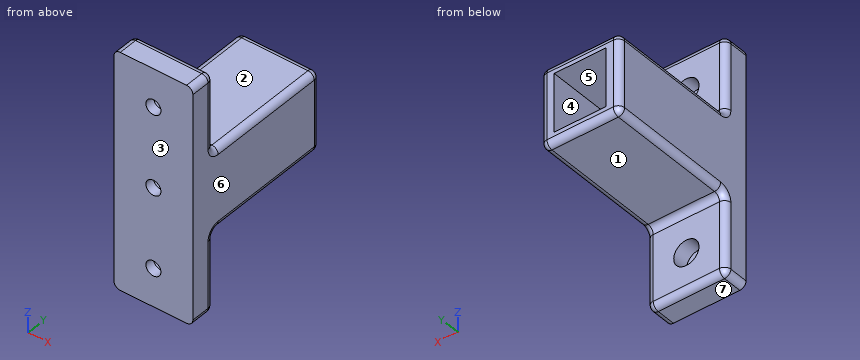
from build123d import *

# Parameters (mm, degrees)
SKETCH1_W               = 25
SKETCH1_H               = 25
SKETCH1_W_2             = 16.4
SKETCH1_H_2             = 18.5
BOSS_EXTRUDE1_DEPTH     = 50
SKETCH6_W               = 25
SKETCH6_H               = 75
BOSS_EXTRUDE3_DEPTH     = 8
FILLET2_R               = 2
SKETCH7_R               = 4
CUT_EXTRUDE1_DEPTH      = 5
CUT_EXTRUDE4_DEPTH      = 64.73774392
CUT_EXTRUDE4_DEPTH_BACK = 64.73774392
SKETCH8_R               = 2.38125


with BuildPart() as part:
    # Sketch1 → Boss-Extrude1 (new body)
    with BuildSketch(Plane(origin=(0, 0, 0), x_dir=(1, 0, 0), z_dir=(0, 1, 0))):
        Rectangle(SKETCH1_W, SKETCH1_H)
        Rectangle(SKETCH1_W_2, SKETCH1_H_2, mode=Mode.SUBTRACT)
    extrude(amount=BOSS_EXTRUDE1_DEPTH)

    # Sketch6 → Boss-Extrude3 (add)
    with BuildSketch(Plane(origin=(0, 0, 0), x_dir=(1, 0, 0), z_dir=(0, 1, 0))):
        Rectangle(SKETCH6_W, SKETCH6_H)
    extrude(amount=BOSS_EXTRUDE3_DEPTH)

    # Fillet2
    fillet2_edges = [part.edges().sort_by_distance(p)[0] for p in [
        (-12.5, 50, 0),
        (0, 50, 12.5),
        (12.5, 4, 37.5),
        (-12.5, 4, -37.5),
        (-12.5, 8, -25),
        (0, 8, -12.5),
        (12.5, 8, -25),
        (0, 8, -37.5),
        (12.5, 8, 25),
        (0, 8, 12.5),
        (-12.5, 8, 25),
        (0, 8, 37.5),
        (12.5, 4, -37.5),
        (-12.5, 4, 37.5),
        (12.5, 50, 0),
        (12.5, 29, 12.5),
        (-12.5, 29, 12.5),
        (-12.5, 29, -12.5),
        (12.5, 29, -12.5),
        (0, 50, -12.5),
    ]]
    fillet(fillet2_edges, radius=FILLET2_R)

    # Sketch7 → Cut-Extrude1 (cut)
    with BuildSketch(Plane(origin=(0, 8, 0), x_dir=(1, 0, 0), z_dir=(0, 1, 0))):
        with Locations(Location((0, 0, 0), (0, 0, 270))):
            Circle(SKETCH7_R)
        with Locations(Location((0, 25.4, 0), (0, 0, 270))):
            Circle(SKETCH7_R)
        with Locations(Location((0, -25.4, 0), (0, 0, 270))):
            Circle(SKETCH7_R)
    extrude(amount=-CUT_EXTRUDE1_DEPTH, mode=Mode.SUBTRACT)

    # Sketch8 → Cut-Extrude4 (cut, two sides: drawn at the far end of the back side and taken through both)
    with BuildSketch(Plane(origin=(0, 0, 0), x_dir=(1, 0, 0), z_dir=(0, 1, 0)).offset(-CUT_EXTRUDE4_DEPTH_BACK)):
        with Locations(Location((0, 0, 0), (0, 0, 270))):
            Circle(SKETCH8_R)
        with Locations(Location((0, 25.4, 0), (0, 0, 270))):
            Circle(SKETCH8_R)
        with Locations(Location((0, -25.4, 0), (0, 0, 270))):
            Circle(SKETCH8_R)
    extrude(amount=CUT_EXTRUDE4_DEPTH + CUT_EXTRUDE4_DEPTH_BACK, mode=Mode.SUBTRACT)


solid = part.part
CAD build for the part. Positions are in the model's coordinates, mm. Face numbers are marked on the shaded views. A direction names the side the tool comes from. Coordinates: 2 decimals unless noted, no trailing zeros. Loops run counter-clockwise (first coordinate to the right, second up) from the corner with the lowest first, then second, coordinate; pieces in that order, holes last. Notation, with made-up numbers: (-1, -19) - (57, -19) arc R21 cw to (57, 19) - close; hole circle Ø6 at (-22, 2). An arc over 180 degrees is marked (long way). Use one line per item in the form item = value. Start each with the question number.
1) Band-saw the part on A-A (y = 24). Give the cut face in (x, z), and give its area (3 significant figures).
2) Band-saw the part on B-B (z = 0). Give the cut face in (x, y).
3) Two-plate mould, pull along X, no slides. Class the marked faces 4, 5, 6 and 7: +X half, -X half, draft (parallel to the pull), parting line (faces both ways), or undercut.
4) Tool access for the marked faces 1, 2 and 3: list every direction of +Z, -Z, +X, -X, +Y, -Y with a clear straight run to the whole face (end or side of a thin tool).
5) Band-saw the part on D-D (z = -18.5). Give the cut face in (x, y), and give its area (3 significant figures).
6) Flat gauge pins, fed straight in: pin 1 (2 mm diameter, centred on x = 7.5, y = 30, fed in from +Z); pin 2 (5 mm diameter, centred on x = 2.5, y = 27, fed in from -Z); pin 3 (6.5 mm diameter, centred on x = -1.5, z = -26, fed in from +Y). Where does each tip first touch, or does it go through?
7) Band-saw the part on C-C (x = 7.25). Give the cut face in (y, z), and give its area (3 significant figures).
8) Drill centre lines: L1, parallel to X at y = 29.5, z = -3.5; L2, parallel to Z at x = 7.25, y = 26.5; L3, parallel to X at y = 2.4, z = -25.4. Where is each one in solid material? Low to high. Write a range as from..to.
Check values:
q1.outline = (-12.5, -10.5) arc R2 ccw to (-10.5, -12.5) - (10.5, -12.5) arc R2 ccw to (12.5, -10.5) - (12.5, 10.5) arc R2 ccw to (10.5, 12.5) - (-10.5, 12.5) arc R2 ccw to (-12.5, 10.5) - close; hole (-8.2, -9.25) - (8.2, -9.25) - (8.2, 9.25) - (-8.2, 9.25) - close
q1.area = 318 mm2
q2.outline = (-12.5, 0) - (-2.38, 0) - (-2.38, 3) - (-4, 3) - (-4, 8) - (-8.2, 8) - (-8.2, 50) - (-10.5, 50) arc R2 ccw to (-12.5, 48) - close; (2.38, 0) - (12.5, 0) - (12.5, 48) arc R2 ccw to (10.5, 50) - (8.2, 50) - (8.2, 8) - (4, 8) - (4, 3) - (2.38, 3) - close
q3.face_4 = undercut
q3.face_5 = undercut
q3.face_6 = +X half
q3.face_7 = draft
q4.face_1 = -Z, +X, -X, +Y
q4.face_2 = +Z, +X, -X, +Y
q4.face_3 = +Z, -Z, +X, -X, -Y
q5.outline = (-12.5, 0) - (12.5, 0) - (12.5, 6) arc R2 ccw to (10.5, 8) - (-10.5, 8) arc R2 ccw to (-12.5, 6) - close
q5.area = 198 mm2
q6.pin_1 = 12.5
q6.pin_2 = -12.5
q6.pin_3 = 8
q7.outline = (0, -37.5) - (6, -37.5) arc R2 ccw to (8, -35.5) - (8, -14.5) arc R2 cw to (10, -12.5) - (48, -12.5) arc R2 ccw to (50, -10.5) - (50, -9.25) - (8, -9.25) - (8, 9.25) - (50, 9.25) - (50, 10.5) arc R2 ccw to (48, 12.5) - (10, 12.5) arc R2 cw to (8, 14.5) - (8, 35.5) arc R2 ccw to (6, 37.5) - (0, 37.5) - close
q7.area = 871 mm2
q8.L1 = -12.5..-8.2, 8.2..12.5
q8.L2 = -12.5..-9.25, 9.25..12.5
q8.L3 = -12.5..-2.38, 2.38..12.5
